CAD build for the part. Positions are in the model's coordinates, mm. Coordinates: 2 decimals unless noted, no trailing zeros. Loops run counter-clockwise (first coordinate to the right, second up) from the corner with the lowest first, then second, coordinate; pieces in that order, holes last. Notation, with made-up numbers: (72.5, -2) -> (127.5, -2) arc R8 ccw to (127.5, 10) -> close; hole circle Ø5 at (13, 85). An arc over 180 degrees is marked (long way). Write item = value, one per line. Start each with the question number.
(1) Drill centre lines: line 1 (Z direction, x = 3.25, y = -230); line 2 (Y direction, x = 4.85, z = -10); line 3 (Y direction, x = 2, z = -305). Where is each one in solid material? Low to high. Write a range as from..to.
(2) Flat gauge pins, fed straight in: P1, Ø1.5, axis at x = 2.5, z = -200.5, coming from the +Y side; P2, Ø1.8, axis at x = 3, z = -27.5, coming from the +Y side. Where does each tip first touch, or does it go through?
(3) Band-saw the part on C-C (z = 0.5). Write the cut outline in (x, y).
(4) Band-saw the part on B-B (x = 3.65). Write the cut outline in (y, z).
(5) Pull direction Z, two halves, no side cores. Call faces 1 (the face through (2.96, -170.04, -71.05)), 2 (the face through (3.04, -8.43, -4.38)), 3 (the face through (2.96, 42.7, -7.05)), 4 (the face through (0, -131, -28)): +Z half, -Z half, draft (parallel to the pull), parting line (faces both ways), or undercut.
(6) Band-saw the part on D-D (z = -173.5). Write the cut outline in (x, y).
(7) Band-saw the part on A-A (y = 0). Write the cut outline in (x, z).
```python
from build123d import *

# Parameters (mm, degrees)
SKETCH1_R           = 4
BOSS_EXTRUDE1_DEPTH = 6
CUT_EXTRUDE1_REACH  = 8
SKETCH3_R           = 9.5
SKETCH4_W           = 50
SKETCH4_H           = 300
BOSS_EXTRUDE2_DEPTH = 6
CUT_EXTRUDE2_REACH  = 8
SKETCH5_R           = 2


with BuildPart() as part:
    # Sketch1 → Boss-Extrude1 (new body)
    with BuildSketch(Plane(origin=(0, 0, 0), x_dir=(0, 0, -1), z_dir=(1, 0, 0))):
        with BuildLine():
            Line((-80, -190), (-80, -250))
            Line((-80, -250), (320, -250))
            Line((320, -250), (320, -190))
            Line((320, -190), (120, -190))
            ThreePointArc((120, -190), (70.502525317, -169.497474683), (50, -120))
            Line((50, -120), (50, 50))
            Line((50, 50), (39, 50))
            Line((39, 50), (39, 43))
            Line((39, 43), (19, 43))
            Line((19, 43), (19, 50))
            Line((19, 50), (-30, 50))
            Line((-30, 50), (-30, -120.049643139))
            ThreePointArc((-30, -120.049643139), (-43.785205981, -163.041073753), (-80, -190))
        make_face()
        with Locations((10, -40)):
            Circle(SKETCH1_R, mode=Mode.SUBTRACT)
        Circle(SKETCH1_R, mode=Mode.SUBTRACT)
        with Locations((10, 40)):
            Circle(SKETCH1_R, mode=Mode.SUBTRACT)
    extrude(amount=BOSS_EXTRUDE1_DEPTH)

    # Sketch3 → Cut-Extrude1 (cut, up to next)
    with BuildSketch(Plane(origin=(6, 0, 0), x_dir=(0, 0, -1), z_dir=(1, 0, 0)), mode=Mode.PRIVATE) as cut_extrude1_sk1:
        Circle(SKETCH3_R)
    cut_extrude1_tool1 = extrude(cut_extrude1_sk1.sketch, amount=-CUT_EXTRUDE1_REACH, mode=Mode.PRIVATE) & part.part
    add(cut_extrude1_tool1.solids().sort_by_distance((6, 0, 0))[0], mode=Mode.SUBTRACT)

    # Sketch4 → Boss-Extrude2 (add)
    with BuildSketch(Plane.ZY):
        with Locations((55, -100)):
            Rectangle(SKETCH4_W, SKETCH4_H)
    extrude(amount=-BOSS_EXTRUDE2_DEPTH)

    # Sketch5 → Cut-Extrude2 (cut, up to next)
    with BuildSketch(Plane.ZY, mode=Mode.PRIVATE) as cut_extrude2_sk1:
        with Locations((65, -210)):
            Circle(SKETCH5_R)
    cut_extrude2_tool1 = extrude(cut_extrude2_sk1.sketch, amount=-CUT_EXTRUDE2_REACH, mode=Mode.PRIVATE) & part.part
    add(cut_extrude2_tool1.solids().sort_by_distance((0, -210, 65))[0], mode=Mode.SUBTRACT)
    # Sketch5 → Cut-Extrude2 (cut, up to next)
    with BuildSketch(Plane.ZY, mode=Mode.PRIVATE) as cut_extrude2_sk2:
        with Locations((65, -230)):
            Circle(SKETCH5_R)
    cut_extrude2_tool2 = extrude(cut_extrude2_sk2.sketch, amount=-CUT_EXTRUDE2_REACH, mode=Mode.PRIVATE) & part.part
    add(cut_extrude2_tool2.solids().sort_by_distance((0, -230, 65))[0], mode=Mode.SUBTRACT)
    # Sketch5 → Cut-Extrude2 (cut, up to next)
    with BuildSketch(Plane.ZY, mode=Mode.PRIVATE) as cut_extrude2_sk3:
        with Locations((-305, -230)):
            Circle(SKETCH5_R)
    cut_extrude2_tool3 = extrude(cut_extrude2_sk3.sketch, amount=-CUT_EXTRUDE2_REACH, mode=Mode.PRIVATE) & part.part
    add(cut_extrude2_tool3.solids().sort_by_distance((0, -230, -305))[0], mode=Mode.SUBTRACT)
    # Sketch5 → Cut-Extrude2 (cut, up to next)
    with BuildSketch(Plane.ZY, mode=Mode.PRIVATE) as cut_extrude2_sk4:
        with Locations((-305, -210)):
            Circle(SKETCH5_R)
    cut_extrude2_tool4 = extrude(cut_extrude2_sk4.sketch, amount=-CUT_EXTRUDE2_REACH, mode=Mode.PRIVATE) & part.part
    add(cut_extrude2_tool4.solids().sort_by_distance((0, -210, -305))[0], mode=Mode.SUBTRACT)


solid = part.part
```
Findings below:
q1.line_1 = -320..-307, -303..63, 67..80
q1.line_2 = -250..-44, -36..36, 44..50
q1.line_3 = -250..-232, -228..-212, -208..-190
q2.P1 = -190
q2.P2 = 43
q3.outline = (0, -250) -> (6, -250) -> (6, -9.49) -> (0, -9.49) -> close; (0, 9.49) -> (6, 9.49) -> (6, 50) -> (0, 50) -> close
q4.outline = (-250, -320) -> (-190, -320) -> (-190, -120) arc R70 cw to (-120, -50) -> (50, -50) -> (50, -39) -> (43, -39) -> (43, -19) -> (50, -19) -> (50, 80) -> (-250, 80) -> close; hole circle Ø4 at (-230, -305); hole circle Ø4 at (-230, 65); hole circle Ø4 at (-210, -305); hole circle Ø4 at (-210, 65); hole circle Ø8 at (-40, -10); hole circle Ø19 at (0, 0); hole circle Ø8 at (40, -10)
q5.face_1 = -Z half
q5.face_2 = undercut
q5.face_3 = undercut
q5.face_4 = draft
q6.outline = (0, -250) -> (6, -250) -> (6, -190) -> (0, -190) -> close
q7.outline = (0, -50) -> (6, -50) -> (6, -9.5) -> (0, -9.5) -> close; (0, 9.5) -> (6, 9.5) -> (6, 80) -> (0, 80) -> close
